For this review, take the finished solid that the model builds, in its own axes (mm). Coordinates: 2 decimals unless noted, no trailing zeros. Order: outer loops, then holes, each group sorted by start corner. A loop starts at its lowest first (then second) coordinate and runs counter-clockwise, first axis right, second up. Notation, with made-up numbers: (-39.5, 62.25) -> (-15.5, 62.25) arc R14 ccw to (-15.5, 81.25) -> close; hole circle Ø9 at (47.5, -22.75). An arc over 180 degrees is marked (long way). Answer as a JSON object with one key per item and string values. Group by question number.
1) Add section A-A, the plane z = 0. Write out the cut boundary in (x, y), then the cut area to 3 significant figures.
2) Draft analysis for pull direction Z (two halves, no side actions). For faces 1 (the conical face through (-13.26, -4.12, -0.91)), 2 (the cylindrical face through (-0.21, -2.77, -1.15)), state which applies: +Z half, -Z half, draft (parallel to the pull), parting line (faces both ways), or undercut.
3) Add section C-C, the plane x = -13. Write out the cut boundary in (y, z).
4) Wall thickness on L1, parallel to Y at x = 5.5, z = 8.25; L2, parallel to Y at x = -3, z = 0; L3, parallel to Z at x = -7, y = 0: over which ranges is each line inside the solid? List them lowest first.
5) For pin 1 (3 mm diameter, centred on x = -8.5, z = 0, fed in from -Y); pin 2 (5 mm diameter, centred on y = -6, z = 4.5, fed in from +X); pin 3 (5 mm diameter, centred on x = 1.5, z = -5.5, fed in from -Y), all flat-tipped, find the tip position at first contact; note any pin that passes through.
6) Add section D-D, the plane x = -0.75. Write out the cut boundary in (y, z), then the cut area to 3 significant figures.
from build123d import *

# Parameters (mm, degrees)
F3_R     = 3
F4_DEPTH = 30.001


with BuildPart() as f1:
    # F0 (on Front) → F1 (revolve)
    with BuildSketch(Plane.XZ):
        Polygon((0, 10), (0, 0), (15, 0), (15, 3), (5, 10), align=None)
    revolve(axis=Axis((7.5, 0, 0), (-1, 0, 0)))

    # F2: F1 across plane


with BuildPart() as f1_1:
    add(f1.part)
    add(f1.part.mirror(Plane.YZ))

    # F3 (on face) → F4 (cut, through all)
    with BuildSketch(Plane(origin=(-15, 0, 0), x_dir=(0, -1, 0), z_dir=(-1, 0, 0))):
        Circle(F3_R)
    extrude(amount=-F4_DEPTH, mode=Mode.SUBTRACT)


solid = f1_1.part
Output values:
{
 "1": {"outline": "(-15, -3) -> (-5, -10) -> (5, -10) -> (15, -3) -> close; (-15, 3) -> (15, 3) -> (5, 10) -> (-5, 10) -> close", "area": "280 mm²"},
 "2": {"face 1": "parting line", "face 2": "undercut"},
 "3": {"outline": "circle Ø8.8 at (0, 0); hole circle Ø6 at (0, 0)"},
 "4": {"L1": "y = -5.01 to 5.01", "L2": "y = -10 to -3, 3 to 10", "L3": "z = -8.6 to -3, 3 to 8.6"},
 "5": {"pin 1": "stops at y = -8.6", "pin 2": "stops at x = 12.14", "pin 3": "stops at y = -9.54"},
 "6": {"outline": "circle Ø20 at (0, 0); hole circle Ø6 at (0, 0)", "area": "286 mm²"}
}
